Input: dimensioned drawing with shaded views. Units: mm. Origin: part minimum x, y, z. A direction names the side the tool comes from. Coordinates: 2 decimals unless noted, no trailing zeros. Write each loop counter-clockwise with the first axis right and the second up, starting at its lowest first coordinate (ties: lowest second). Pieces come first, ordered by that corner, then holes. Notation, with made-up numbers: (20, 6.5) -> (37, 6.5) arc R29 cw to (37, 43.5) -> close; hole circle Ø2 at (-13.5, 74.25). An arc over 180 degrees is marked (long way). One line per item, written item: value. Start each with the question number.
1. Section query B-B, the plane y = 5. Output: boundary loops of the cut face in (x, z), and give its area (3 significant figures).
2. Section query A-A, the plane x = 6. Output: boundary loops of the cut face in (y, z).
3. Section query D-D, the plane x = 2.5. Output: boundary loops of the cut face in (y, z).
4. First-contact query: P1, Ø1.3, axis at x = 6, z = 6.5, coming from the +Y side. Flat tip, straight axial feed; report the tip coordinate or a pass-through.
5. Section query C-C, the plane z = 3. Output: boundary loops of the cut face in (x, y).
6. Access query for the marked faces 1 and 2. Directions: +Z, -Z, +X, -X, +Y, -Y. A direction counts if a zero-diameter tool reaches every point of the face in a straight line with its end or side. Return the directions, or none.
7. Line query: line 1 (Z direction, x = 6.75, y = 7); line 2 (Y direction, x = 11.25, z = 26.5); line 3 (X direction, y = 4.75, z = 2.5). Output: solid intervals per line, ascending.
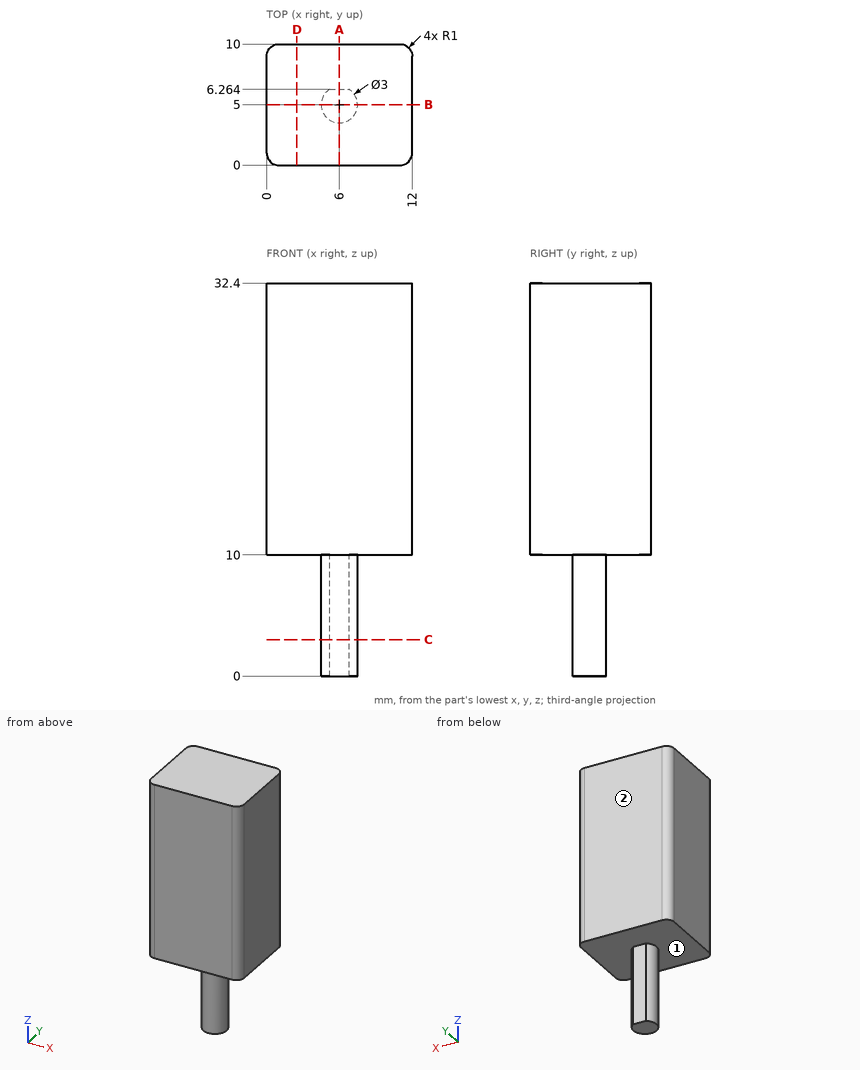
Computed values:
1. outline: (0, 10) -> (4.5, 10) -> (4.5, 0) -> (7.5, 0) -> (7.5, 10) -> (12, 10) -> (12, 32.4) -> (0, 32.4) -> close
1. area: 299 mm²
2. outline: (0, 10) -> (3.5, 10) -> (3.5, 0) -> (6.26, 0) -> (6.26, 10) -> (10, 10) -> (10, 32.4) -> (0, 32.4) -> close
3. outline: (0, 10) -> (10, 10) -> (10, 32.4) -> (0, 32.4) -> close
4. P1: stops at y = 6.26
5. outline: (5.19, 6.26) arc R1.5 ccw (long way) to (6.81, 6.26) -> close
6. face 1: -Z
6. face 2: +Z, -Z, +X, -X, +Y
7. line 1: z = 10 to 32.4
7. line 2: y = 0.03 to 9.97
7. line 3: x = 4.52 to 7.48
